from build123d import *

# Parameters (mm, degrees)
SKETCH_1_W          = 60.5
SKETCH_1_H          = 95.5
EXTRUDE_1_DEPTH     = 16.2
SKETCH_2_R          = 6
SKETCH_2_R_2        = 4
SKETCH_2_R_3        = 2
EXTRUDE_2_DEPTH     = 7
EXTRUDE_START       = 6
SKETCH_7_R          = 6
EXTRUDE_6_DEPTH     = 6
SKETCH_3_R          = 4
EXTRUDE_3_DEPTH     = 30
CUT_EXTRUDE_START   = -16
CUT_EXTRUDE_1_DEPTH = 16
SKETCH_5_R          = 4
SKETCH_5_R_2        = 2
EXTRUDE_4_DEPTH     = 8
SKETCH_6_R          = 18
EXTRUDE_5_DEPTH     = 57.6


with BuildPart() as part:
    # 草图1 → 凸台-拉伸1 (new body)
    with BuildSketch(Plane(origin=(0, 0, 0), x_dir=(1, 0, 0), z_dir=(0, 1, 0))):
        with Locations((0, -23.75)):
            Rectangle(SKETCH_1_W, SKETCH_1_H)
    extrude(amount=EXTRUDE_1_DEPTH)

    # 草图2 → 凸台-拉伸2 (add)
    # profile 1 of 5: a face of its own
    with BuildSketch(Plane(origin=(0, 16.2, 0), x_dir=(1, 0, 0), z_dir=(0, 1, 0))):
        with Locations(Location((0, 0, 0), (0, 0, 90))):
            Circle(SKETCH_2_R)
    # profile 2 of 5: a face of its own
    with BuildSketch(Plane(origin=(0, 16.2, 0), x_dir=(1, 0, 0), z_dir=(0, 1, 0))):
        with Locations(Location((-20, 0, 0), (0, 0, 90))):
            Circle(SKETCH_2_R_2)
        with Locations(Location((-20, 0, 0), (0, 0, 270))):
            Circle(SKETCH_2_R_3, mode=Mode.SUBTRACT)
    # profile 3 of 5: a face of its own
    with BuildSketch(Plane(origin=(0, 16.2, 0), x_dir=(1, 0, 0), z_dir=(0, 1, 0))):
        with Locations(Location((20, 0, 0), (0, 0, 90))):
            Circle(SKETCH_2_R_2)
        with Locations(Location((20, 0, 0), (0, 0, 270))):
            Circle(SKETCH_2_R_3, mode=Mode.SUBTRACT)
    # profile 4 of 5: a face of its own
    with BuildSketch(Plane(origin=(0, 16.2, 0), x_dir=(1, 0, 0), z_dir=(0, 1, 0))):
        with Locations(Location((20, -40, 0), (0, 0, 90))):
            Circle(SKETCH_2_R_2)
        with Locations(Location((20, -40, 0), (0, 0, 270))):
            Circle(SKETCH_2_R_3, mode=Mode.SUBTRACT)
    # profile 5 of 5: a face of its own
    with BuildSketch(Plane(origin=(0, 16.2, 0), x_dir=(1, 0, 0), z_dir=(0, 1, 0))):
        with Locations(Location((-20, -40, 0), (0, 0, 90))):
            Circle(SKETCH_2_R_2)
        with Locations(Location((-20, -40, 0), (0, 0, 270))):
            Circle(SKETCH_2_R_3, mode=Mode.SUBTRACT)
    extrude(amount=EXTRUDE_2_DEPTH)

    # 草图7 → 凸台-拉伸6 (add)
    with BuildSketch(Plane.XZ.offset(EXTRUDE_START)):
        with Locations(Location((0, 0, 0), (0, 0, 270))):
            Circle(SKETCH_7_R)
    extrude(amount=-EXTRUDE_6_DEPTH)

    # 草图3 → 凸台-拉伸3 (add)
    with BuildSketch(Plane(origin=(0, -6, 0), x_dir=(1, 0, 0), z_dir=(0, 1, 0))):
        with Locations(Location((0, 0, 0), (0, 0, 270))):
            Circle(SKETCH_3_R)
    extrude(amount=-EXTRUDE_3_DEPTH)

    # 草图4 → 切除-拉伸1 (cut)
    with BuildSketch(Plane(origin=(0, -36, 0), x_dir=(-1, 0, 0), z_dir=(0, -1, 0)).offset(CUT_EXTRUDE_START)):
        with BuildLine():
            Line((-3.464101615, -2), (3.464101615, -2))
            ThreePointArc((3.464101615, -2), (0, -4), (-3.464101615, -2))
        make_face()
    extrude(amount=CUT_EXTRUDE_1_DEPTH, mode=Mode.SUBTRACT)

    # 草图5 → 凸台-拉伸4 (add)
    # profile 1 of 4: a face of its own
    with BuildSketch(Plane(origin=(0, 0, 0), x_dir=(-1, 0, 0), z_dir=(0, -1, 0))):
        with Locations(Location((-17.5, 12.5, 0), (0, 0, 90))):
            Circle(SKETCH_5_R)
        with Locations(Location((-17.5, 12.5, 0), (0, 0, 90))):
            Circle(SKETCH_5_R_2, mode=Mode.SUBTRACT)
    # profile 2 of 4: a face of its own
    with BuildSketch(Plane(origin=(0, 0, 0), x_dir=(-1, 0, 0), z_dir=(0, -1, 0))):
        with Locations(Location((17.5, 12.5, 0), (0, 0, 90))):
            Circle(SKETCH_5_R)
        with Locations(Location((17.5, 12.5, 0), (0, 0, 90))):
            Circle(SKETCH_5_R_2, mode=Mode.SUBTRACT)
    # profile 3 of 4: a face of its own
    with BuildSketch(Plane(origin=(0, 0, 0), x_dir=(-1, 0, 0), z_dir=(0, -1, 0))):
        with Locations(Location((17.5, -12.5, 0), (0, 0, 90))):
            Circle(SKETCH_5_R)
        with Locations(Location((17.5, -12.5, 0), (0, 0, 90))):
            Circle(SKETCH_5_R_2, mode=Mode.SUBTRACT)
    # profile 4 of 4: a face of its own
    with BuildSketch(Plane(origin=(0, 0, 0), x_dir=(-1, 0, 0), z_dir=(0, -1, 0))):
        with Locations(Location((-17.5, -12.5, 0), (0, 0, 90))):
            Circle(SKETCH_5_R)
        with Locations(Location((-17.5, -12.5, 0), (0, 0, 90))):
            Circle(SKETCH_5_R_2, mode=Mode.SUBTRACT)
    extrude(amount=EXTRUDE_4_DEPTH)

    # 草图6 → 凸台-拉伸5 (add)
    with BuildSketch(Plane.XZ):
        with Locations(Location((0, 53.5, 0), (0, 0, 90))):
            Circle(SKETCH_6_R)
    extrude(amount=EXTRUDE_5_DEPTH)


solid = part.part
Build history of the part. All positions in model axes, mm. A direction names the side the tool comes from. Round coordinates to 2 decimals unless told otherwise and drop trailing zeros. Write each loop counter-clockwise with the first axis right and the second up, starting at its lowest first coordinate (ties: lowest second). Pieces come first, ordered by that corner, then holes. Notation, with made-up numbers: (82.5, 77) - (97.5, 77) arc R31 ccw to (97.5, 105) - close; hole circle Ø10 at (48, 9). An arc over 180 degrees is marked (long way). One line per question, with ' | ' between items.
1. Band-saw the part on A-A, the plane z = 53.5. Write the cut outline in (x, y).
Results are:
outline: (-30.25, 0) - (-18, 0) - (-18, -57.6) - (18, -57.6) - (18, 0) - (30.25, 0) - (30.25, 16.2) - (-30.25, 16.2) - close
2. Band-saw the part on D-D, the plane y = -42. Write the cut outline in (x, z), and give its area (3 significant figures).
Results are:
outline: circle Ø36 at (0, 53.5) | area: 1,020 mm^2
3. Band-saw the part on B-B, the plane y = -11. Write the cut outline in (x, z).
Results are:
outline: circle Ø36 at (0, 53.5); circle Ø8 at (0, 0)
4. Drill centre lines: line 1 along X through (y, z) = (21, 40); line 2 along Y through (x, z) = (-5, 56); line 3 along Y through (x, z) = (12, 15). Where is each one in solid material? Low to high. Write a range as from..to.
Results are:
line 1: -24..-22, -18..-16, 16..18, 22..24 | line 2: -57.6..16.2 | line 3: 0..16.2
5. Mould opens along Z. For faces 1 (the face through (21, 23.2, 2)), 2 (the face through (-14.8, -3.94, 15.45)), 3 (the face through (-18, 0, -13)) say: released by +Z, released by -Z, zero draft, split by the parting line, or undercut.
Results are:
face 1: zero draft | face 2: undercut | face 3: undercut
6. Tool access for faces 4 (the face through (30.25, 8, 24)), 5 (the face through (16.034, 19.651, 0.521)), 6 (the face through (0, -36, 0)), 7 (the face through (-2.4, -20.8, -3.2)), 8 (the face through (0, -28, 2)): list every direction of +Z, -Z, +X, -X, +Y, -Y with a clear straight run to the whole face (end or side of a thin tool).
Results are:
face 4: +Z, -Z, +X, +Y, -Y | face 5: +Y | face 6: -Z, +X, -X, -Y | face 7: -Y | face 8: +X, -X, -Y
7. Drop flat-ended pins along their axis: pin 1 Ø5 at (x, z) = (12, 45) entering from +Y; pin 2 Ø4.5 at (x, z) = (-20, 0) entering from -Y; pin 3 Ø9 at (x, z) = (19, -12) entering from -Y; pin 4 Ø2 at (y, z) = (-35.5, 33.5) entering from -X. Give the stop position or say it passes through.
Results are:
pin 1: y = 16.2 | pin 2: y = 0 | pin 3: y = -8 | pin 4: through
